The model under review builds one solid part; all positions refer to its coordinate system, in mm. Coordinates: 2 decimals unless noted, no trailing zeros. Loops run counter-clockwise (first coordinate to the right, second up) from the corner with the lowest first, then second, coordinate; pieces in that order, holes last. Notation, with made-up numbers: (74.5, -16.5) - (93.5, -16.5) arc R8 ccw to (93.5, -7.5) - close; hole circle Ø3 at (34, 86.25). An arc over 180 degrees is marked (long way). Use a Markdown table: item, result. Add a question column.
1) The part is to be moulded in two halves that separate along Y. For faces 1 (the flat face through (104, 26, 0)), 2 (the flat face through (131, 11, 2.54)), 3 (the flat face through (104, 0, 6)), say which applies: pulls with the +Y half, pulls with the -Y half, needs draft (parallel to the pull), parting line crosses it, or undercut.
2) Add section B-B, the plane z = 8.75. Give the number of separate pieces and of enclosed holes in the cut face, and give its area (3 significant figures).
3) To check wall thickness, follow L1, parallel to Y at x = 29, z = 5.5; L2, parallel to X at y = 44.5, z = 11.25; L3, parallel to Y at x = 20, z = 12. State the ranges of each line that lie inside material, in increasing order. Write a range as [from, to].
4) Add section A-A, the plane x = 41.5. Give the boundary of the cut face in (y, z).
```python
from build123d import *

# Parameters (mm, degrees)
F0_W     = 210.82
F0_H     = 50.8
F1_DEPTH = 12.7
F3_DEPTH = 10.16


with BuildPart() as f1:
    # F0 (on Top) → F1 (new body)
    with BuildSketch(Plane.XY):
        with Locations((105.41, 25.4)):
            Rectangle(F0_W, F0_H)
    extrude(amount=F1_DEPTH)

    # F2 (on face) → F3 (cut)
    with BuildSketch(Plane.XY.offset(12.7)):
        with BuildLine():
            ThreePointArc((8.332038, 43.737962), (6.255988, 44.150914), (5.08, 42.390923))
            Line((5.08, 42.390923), (5.08, 8.409077))
            ThreePointArc((5.08, 8.409077), (6.255988, 6.649086), (8.332038, 7.062038))
            Line((8.332038, 7.062038), (25.322962, 24.052962))
            ThreePointArc((25.322962, 24.052962), (25.880923, 25.4), (25.322962, 26.747038))
            Line((25.322962, 26.747038), (8.332038, 43.737962))
        make_face()
        with BuildLine():
            Line((50.087962, 43.737962), (33.097038, 26.747038))
            ThreePointArc((33.097038, 26.747038), (32.539077, 25.4), (33.097038, 24.052962))
            Line((33.097038, 24.052962), (50.087962, 7.062038))
            ThreePointArc((50.087962, 7.062038), (52.164012, 6.649086), (53.34, 8.409077))
            Line((53.34, 8.409077), (53.34, 42.390923))
            ThreePointArc((53.34, 42.390923), (52.164012, 44.150914), (50.087962, 43.737962))
        make_face()
        with BuildLine():
            ThreePointArc((60.402038, 43.737962), (58.325988, 44.150914), (57.15, 42.390923))
            Line((57.15, 42.390923), (57.15, 8.409077))
            ThreePointArc((57.15, 8.409077), (58.325988, 6.649086), (60.402038, 7.062038))
            Line((60.402038, 7.062038), (77.392962, 24.052962))
            ThreePointArc((77.392962, 24.052962), (77.950923, 25.4), (77.392962, 26.747038))
            Line((77.392962, 26.747038), (60.402038, 43.737962))
        make_face()
        with BuildLine():
            Line((104.14, 8.409077), (104.14, 42.390923))
            ThreePointArc((104.14, 42.390923), (102.964012, 44.150914), (100.887962, 43.737962))
            Line((100.887962, 43.737962), (83.897038, 26.747038))
            ThreePointArc((83.897038, 26.747038), (83.339077, 25.4), (83.897038, 24.052962))
            Line((83.897038, 24.052962), (100.887962, 7.062038))
            ThreePointArc((100.887962, 7.062038), (102.964012, 6.649086), (104.14, 8.409077))
        make_face()
        with BuildLine():
            ThreePointArc((111.202038, 43.737962), (109.125988, 44.150914), (107.95, 42.390923))
            Line((107.95, 42.390923), (107.95, 8.409077))
            ThreePointArc((107.95, 8.409077), (109.125988, 6.649086), (111.202038, 7.062038))
            Line((111.202038, 7.062038), (128.192962, 24.052962))
            ThreePointArc((128.192962, 24.052962), (128.750923, 25.4), (128.192962, 26.747038))
            Line((128.192962, 26.747038), (111.202038, 43.737962))
        make_face()
        with BuildLine():
            Line((154.94, 8.409077), (154.94, 42.390923))
            ThreePointArc((154.94, 42.390923), (153.764012, 44.150914), (151.687962, 43.737962))
            Line((151.687962, 43.737962), (134.697038, 26.747038))
            ThreePointArc((134.697038, 26.747038), (134.139077, 25.4), (134.697038, 24.052962))
            Line((134.697038, 24.052962), (151.687962, 7.062038))
            ThreePointArc((151.687962, 7.062038), (153.764012, 6.649086), (154.94, 8.409077))
        make_face()
        with BuildLine():
            ThreePointArc((162.002038, 43.737962), (159.925988, 44.150914), (158.75, 42.390923))
            Line((158.75, 42.390923), (158.75, 8.409077))
            ThreePointArc((158.75, 8.409077), (159.925988, 6.649086), (162.002038, 7.062038))
            Line((162.002038, 7.062038), (178.992962, 24.052962))
            ThreePointArc((178.992962, 24.052962), (179.550923, 25.4), (178.992962, 26.747038))
            Line((178.992962, 26.747038), (162.002038, 43.737962))
        make_face()
        with BuildLine():
            Line((205.74, 8.409077), (205.74, 42.390923))
            ThreePointArc((205.74, 42.390923), (204.564012, 44.150914), (202.487962, 43.737962))
            Line((202.487962, 43.737962), (185.497038, 26.747038))
            ThreePointArc((185.497038, 26.747038), (184.939077, 25.4), (185.497038, 24.052962))
            Line((185.497038, 24.052962), (202.487962, 7.062038))
            ThreePointArc((202.487962, 7.062038), (204.564012, 6.649086), (205.74, 8.409077))
        make_face()
        with BuildLine():
            Line((44.930923, 46.99), (13.489077, 46.99))
            ThreePointArc((13.489077, 46.99), (11.729086, 45.814012), (12.142038, 43.737962))
            Line((12.142038, 43.737962), (27.862962, 28.017038))
            ThreePointArc((27.862962, 28.017038), (29.21, 27.459077), (30.557038, 28.017038))
            Line((30.557038, 28.017038), (46.277962, 43.737962))
            ThreePointArc((46.277962, 43.737962), (46.690914, 45.814012), (44.930923, 46.99))
        make_face()
        with BuildLine():
            ThreePointArc((12.142038, 7.062038), (11.729086, 4.985988), (13.489077, 3.81))
            Line((13.489077, 3.81), (44.930923, 3.81))
            ThreePointArc((44.930923, 3.81), (46.690914, 4.985988), (46.277962, 7.062038))
            Line((46.277962, 7.062038), (30.557038, 22.782962))
            ThreePointArc((30.557038, 22.782962), (29.21, 23.340923), (27.862962, 22.782962))
            Line((27.862962, 22.782962), (12.142038, 7.062038))
        make_face()
        with BuildLine():
            Line((95.730923, 46.99), (65.559077, 46.99))
            ThreePointArc((65.559077, 46.99), (63.799086, 45.814012), (64.212038, 43.737962))
            Line((64.212038, 43.737962), (79.297962, 28.652038))
            ThreePointArc((79.297962, 28.652038), (80.645, 28.094077), (81.992038, 28.652038))
            Line((81.992038, 28.652038), (97.077962, 43.737962))
            ThreePointArc((97.077962, 43.737962), (97.490914, 45.814012), (95.730923, 46.99))
        make_face()
        with BuildLine():
            ThreePointArc((64.212038, 7.062038), (63.799086, 4.985988), (65.559077, 3.81))
            Line((65.559077, 3.81), (95.730923, 3.81))
            ThreePointArc((95.730923, 3.81), (97.490914, 4.985988), (97.077962, 7.062038))
            Line((97.077962, 7.062038), (81.992038, 22.147962))
            ThreePointArc((81.992038, 22.147962), (80.645, 22.705923), (79.297962, 22.147962))
            Line((79.297962, 22.147962), (64.212038, 7.062038))
        make_face()
        with BuildLine():
            Line((146.530923, 46.99), (116.359077, 46.99))
            ThreePointArc((116.359077, 46.99), (114.599086, 45.814012), (115.012038, 43.737962))
            Line((115.012038, 43.737962), (130.097962, 28.652038))
            ThreePointArc((130.097962, 28.652038), (131.445, 28.094077), (132.792038, 28.652038))
            Line((132.792038, 28.652038), (147.877962, 43.737962))
            ThreePointArc((147.877962, 43.737962), (148.290914, 45.814012), (146.530923, 46.99))
        make_face()
        with BuildLine():
            ThreePointArc((115.012038, 7.062038), (114.599086, 4.985988), (116.359077, 3.81))
            Line((116.359077, 3.81), (146.530923, 3.81))
            ThreePointArc((146.530923, 3.81), (148.290914, 4.985988), (147.877962, 7.062038))
            Line((147.877962, 7.062038), (132.792038, 22.147962))
            ThreePointArc((132.792038, 22.147962), (131.445, 22.705923), (130.097962, 22.147962))
            Line((130.097962, 22.147962), (115.012038, 7.062038))
        make_face()
        with BuildLine():
            Line((197.330923, 46.99), (167.159077, 46.99))
            ThreePointArc((167.159077, 46.99), (165.399086, 45.814012), (165.812038, 43.737962))
            Line((165.812038, 43.737962), (180.897962, 28.652038))
            ThreePointArc((180.897962, 28.652038), (182.245, 28.094077), (183.592038, 28.652038))
            Line((183.592038, 28.652038), (198.677962, 43.737962))
            ThreePointArc((198.677962, 43.737962), (199.090914, 45.814012), (197.330923, 46.99))
        make_face()
        with BuildLine():
            ThreePointArc((165.812038, 7.062038), (165.399086, 4.985988), (167.159077, 3.81))
            Line((167.159077, 3.81), (197.330923, 3.81))
            ThreePointArc((197.330923, 3.81), (199.090914, 4.985988), (198.677962, 7.062038))
            Line((198.677962, 7.062038), (183.592038, 22.147962))
            ThreePointArc((183.592038, 22.147962), (182.245, 22.705923), (180.897962, 22.147962))
            Line((180.897962, 22.147962), (165.812038, 7.062038))
        make_face()
    extrude(amount=-F3_DEPTH, mode=Mode.SUBTRACT)


solid = f1.part
```
From the geometry:
| question | item | result |
|---|---|---|
| 1 | face 1 | needs draft |
| 1 | face 2 | undercut |
| 1 | face 3 | pulls with the -Y half |
| 2 | separate pieces | 1 |
| 2 | enclosed holes | 16 |
| 2 | area | 3,990 mm^2 |
| 3 | L1 | y = [0, 3.81], [23.33, 27.47], [46.99, 50.8] |
| 3 | L2 | x = [0, 11.68], [46.74, 63.75], [97.54, 114.55], [148.34, 165.35], [199.14, 210.82] |
| 3 | L3 | y = [0, 3.81], [14.92, 18.73], [32.07, 35.88], [46.99, 50.8] |
| 4 | outline | (0, 0) - (50.8, 0) - (50.8, 12.7) - (46.99, 12.7) - (46.99, 2.54) - (38.96, 2.54) - (38.96, 12.7) - (35.15, 12.7) - (35.15, 2.54) - (15.65, 2.54) - (15.65, 12.7) - (11.84, 12.7) - (11.84, 2.54) - (3.81, 2.54) - (3.81, 12.7) - (0, 12.7) - close |
